CAD build for the part. Positions are in the model's coordinates, mm. A direction names the side the tool comes from. Coordinates: 2 decimals unless noted, no trailing zeros. Loops run counter-clockwise (first coordinate to the right, second up) from the corner with the lowest first, then second, coordinate; pieces in that order, holes last. Notation, with made-up numbers: (85.5, 34.5) - (115.5, 34.5) arc R34 ccw to (115.5, 65.5) - close; hole circle Ø10 at (41, 63.5). An arc over 180 degrees is marked (long way). Put each result on its own line as item: value.
```python
from build123d import *

# Parameters (mm, degrees)
SKETCH1_W           = 86
SKETCH1_H           = 86
SKETCH1_R           = 1.5
SKETCH1_R_2         = 11.5
SKETCH1_R_3         = 1.75
SKETCH1_W_2         = 9
SKETCH1_H_2         = 24
BOSS_EXTRUDE1_DEPTH = 5
FILLET1_R           = 4
SKETCH2_R           = 1
CUT_EXTRUDE1_DEPTH  = 122.725100123


with BuildPart() as part:
    # Sketch1 → Boss-Extrude1 (new body)
    with BuildSketch(Plane.XY):
        with Locations((43, 43)):
            Rectangle(SKETCH1_W, SKETCH1_H)
        with Locations((25, 61)):
            Circle(SKETCH1_R, mode=Mode.SUBTRACT)
        with Locations((61, 61)):
            Circle(SKETCH1_R, mode=Mode.SUBTRACT)
        with Locations((25, 25)):
            Circle(SKETCH1_R, mode=Mode.SUBTRACT)
        with Locations((61, 25)):
            Circle(SKETCH1_R, mode=Mode.SUBTRACT)
        with Locations((43, 43)):
            Circle(SKETCH1_R_2, mode=Mode.SUBTRACT)
        with Locations((43, 64.920310217)):
            Circle(SKETCH1_R_3, mode=Mode.SUBTRACT)
        with Locations((64.920310217, 43)):
            Circle(SKETCH1_R_3, mode=Mode.SUBTRACT)
        with Locations((43, 21.079689783)):
            Circle(SKETCH1_R_3, mode=Mode.SUBTRACT)
        with Locations((21.079689783, 43)):
            Circle(SKETCH1_R_3, mode=Mode.SUBTRACT)
        with Locations((75, 66)):
            Rectangle(SKETCH1_W_2, SKETCH1_H_2, mode=Mode.SUBTRACT)
        with BuildLine():
            Line((68.5, 66.5), (68.5, 65.5))
            ThreePointArc((68.5, 65.5), (67.5, 64.5), (66.5, 65.5))
            Line((66.5, 65.5), (66.5, 66.5))
            ThreePointArc((66.5, 66.5), (67.5, 67.5), (68.5, 66.5))
        make_face(mode=Mode.SUBTRACT)
        with BuildLine():
            Line((81.5, 66.5), (81.5, 65.5))
            ThreePointArc((81.5, 65.5), (82.5, 64.5), (83.5, 65.5))
            Line((83.5, 65.5), (83.5, 66.5))
            ThreePointArc((83.5, 66.5), (82.5, 67.5), (81.5, 66.5))
        make_face(mode=Mode.SUBTRACT)
        with BuildLine():
            Line((68.5, 19.5), (68.5, 20.5))
            ThreePointArc((68.5, 20.5), (67.5, 21.5), (66.5, 20.5))
            Line((66.5, 20.5), (66.5, 19.5))
            ThreePointArc((66.5, 19.5), (67.5, 18.5), (68.5, 19.5))
        make_face(mode=Mode.SUBTRACT)
        with BuildLine():
            Line((81.5, 19.5), (81.5, 20.5))
            ThreePointArc((81.5, 20.5), (82.5, 21.5), (83.5, 20.5))
            Line((83.5, 20.5), (83.5, 19.5))
            ThreePointArc((83.5, 19.5), (82.5, 18.5), (81.5, 19.5))
        make_face(mode=Mode.SUBTRACT)
        with Locations((75, 20)):
            Rectangle(SKETCH1_W_2, SKETCH1_H_2, mode=Mode.SUBTRACT)
        with BuildLine():
            Line((17.5, 66.5), (17.5, 65.5))
            ThreePointArc((17.5, 65.5), (18.5, 64.5), (19.5, 65.5))
            Line((19.5, 65.5), (19.5, 66.5))
            ThreePointArc((19.5, 66.5), (18.5, 67.5), (17.5, 66.5))
        make_face(mode=Mode.SUBTRACT)
        with BuildLine():
            Line((4.5, 66.5), (4.5, 65.5))
            ThreePointArc((4.5, 65.5), (3.5, 64.5), (2.5, 65.5))
            Line((2.5, 65.5), (2.5, 66.5))
            ThreePointArc((2.5, 66.5), (3.5, 67.5), (4.5, 66.5))
        make_face(mode=Mode.SUBTRACT)
        with BuildLine():
            Line((17.5, 19.5), (17.5, 20.5))
            ThreePointArc((17.5, 20.5), (18.5, 21.5), (19.5, 20.5))
            Line((19.5, 20.5), (19.5, 19.5))
            ThreePointArc((19.5, 19.5), (18.5, 18.5), (17.5, 19.5))
        make_face(mode=Mode.SUBTRACT)
        with BuildLine():
            Line((4.5, 19.5), (4.5, 20.5))
            ThreePointArc((4.5, 20.5), (3.5, 21.5), (2.5, 20.5))
            Line((2.5, 20.5), (2.5, 19.5))
            ThreePointArc((2.5, 19.5), (3.5, 18.5), (4.5, 19.5))
        make_face(mode=Mode.SUBTRACT)
        with Locations((11, 20)):
            Rectangle(SKETCH1_W_2, SKETCH1_H_2, mode=Mode.SUBTRACT)
        with Locations((11, 66)):
            Rectangle(SKETCH1_W_2, SKETCH1_H_2, mode=Mode.SUBTRACT)
    extrude(amount=BOSS_EXTRUDE1_DEPTH)

    # Fillet1
    fillet1_edges = [part.edges().sort_by_distance(p)[0] for p in [
        (0, 86, 2.5),
        (86, 86, 2.5),
        (86, 0, 2.5),
        (0, 0, 2.5),
    ]]
    fillet(fillet1_edges, radius=FILLET1_R)

    # Sketch2 → Cut-Extrude1 (cut, through all)
    with BuildSketch(Plane.XY.offset(5)):
        with Locations((83, 36.4)):
            Circle(SKETCH2_R)
        with Locations((83, 30)):
            Circle(SKETCH2_R)
        with BuildLine():
            Line((33, 9), (53, 9))
            ThreePointArc((53, 9), (56, 6), (53, 3))
            Line((53, 3), (33, 3))
            ThreePointArc((33, 3), (30, 6), (33, 9))
        make_face()
    extrude(amount=-CUT_EXTRUDE1_DEPTH, mode=Mode.SUBTRACT)


solid = part.part
```
Q1. Slice it at A-A, the plane y = 43. Give the cut face in (x, z).
Determined:
outline: (0, 0) - (19.33, 0) - (19.33, 5) - (0, 5) - close; (22.83, 0) - (31.5, 0) - (31.5, 5) - (22.83, 5) - close; (54.5, 0) - (63.17, 0) - (63.17, 5) - (54.5, 5) - close; (66.67, 0) - (86, 0) - (86, 5) - (66.67, 5) - close
Q2. Wall check: L1, parallel to X at y = 71.5, z = 3.9; L2, parallel to Y at x = 43, z = 3.25; L3, parallel to Y at x = 61, z = 2.3. Give the ranges that are in metal, low to high. Write a range as from..to.
Determined:
L1: 0..6.5, 15.5..70.5, 79.5..86
L2: 0..3, 9..19.33, 22.83..31.5, 54.5..63.17, 66.67..86
L3: 0..23.5, 26.5..59.5, 62.5..86
Q3. Slice it at C-C, the plane y = 25. Give the cut face in (x, z), then the cut area to 3 significant figures.
Determined:
outline: (0, 0) - (6.5, 0) - (6.5, 5) - (0, 5) - close; (15.5, 0) - (23.5, 0) - (23.5, 5) - (15.5, 5) - close; (26.5, 0) - (59.5, 0) - (59.5, 5) - (26.5, 5) - close; (62.5, 0) - (70.5, 0) - (70.5, 5) - (62.5, 5) - close; (79.5, 0) - (86, 0) - (86, 5) - (79.5, 5) - close
area: 310 mm2
Q4. Tool access for faces 1 (the flat face through (86, 42, 2)), 2 (the flat face through (11, 32, 2)): list every direction of +Z, -Z, +X, -X, +Y, -Y with a clear straight run to the whole face (end or side of a thin tool).
Determined:
face 1: +Z, -Z, +X, +Y, -Y
face 2: +Z, -Z
Q5. Slice it at B-B, the plane x = 25. Give the cut face in (y, z).
Determined:
outline: (0, 0) - (23.5, 0) - (23.5, 5) - (0, 5) - close; (26.5, 0) - (59.5, 0) - (59.5, 5) - (26.5, 5) - close; (62.5, 0) - (86, 0) - (86, 5) - (62.5, 5) - close
Q6. Slice it at D-D, the plane y = 13. Give the cut face in (x, z), then the cut area to 3 significant figures.
Determined:
outline: (0, 0) - (6.5, 0) - (6.5, 5) - (0, 5) - close; (15.5, 0) - (70.5, 0) - (70.5, 5) - (15.5, 5) - close; (79.5, 0) - (86, 0) - (86, 5) - (79.5, 5) - close
area: 340 mm2
Q7. Pin check, flat tip, straight feed: pin 1 Ø4 at (x, y) = (21.08, 43) entering from +Z. Stop position of the tip, or through.
Determined:
pin 1: z = 5
Q8. Mould opens along X. For faces 3 (the cylindrical face through (84.797, 1.141, 2.535)), 4 (the cylindrical face through (1.141, 84.797, 2.535)), 5 (the flat face through (75, 78, 2)) say: +X half, -X half, draft (parallel to the pull), parting line (faces both ways), or undercut.
Determined:
face 3: +X half
face 4: -X half
face 5: undercut
